Work out the finished part from the listing and answer in its coordinate system (mm). Give positions to 0.01 mm unless a question says otherwise; leave off trailing zeros. Write each loop counter-clockwise with the first axis right and the second up, starting at its lowest first coordinate (ties: lowest second). Pieces come first, ordered by that corner, then holes. Notation, with made-up numbers: (19.5, 29.5) -> (63.5, 29.5) arc R34 ccw to (63.5, 59.5) -> close; hole circle Ø11 at (2, -14.75). An arc over 180 degrees is marked (long way). Use a Markdown table: item, result. Add a question column.
Q1. Section C-C, the plane x = 107 is taken. Give the vertices of the cut face in (y, z), plus the area to 3 significant figures.
Q2. Section B-B, the plane y = 27.5 is taken. Give the vertices of the cut face in (x, z), plus the area to 3 significant figures.
Q3. Consider line 1 (Y direction, x = 18, z = 7.1); line 2 (Y direction, x = 52, z = 7.3); line 3 (X direction, y = 104, z = 8.55). Determine where each line is inside the solid, lowest interval first.
Q4. Section A-A, the plane z = 6.4 is taken. Give the vertices of the cut face in (x, y).
Q5. Each of these flat-tipped pins is pushed along its axis until it touches: pin 1 Ø1 at (y, z) = (102.5, 6) entering from -X; pin 2 Ø2.5 at (y, z) = (27.5, 7) entering from -X; pin 3 Ø5 at (x, y) = (155.28, 47.79) entering from +Z; pin 4 Ø2.5 at (x, z) = (6, 8) entering from -Y. Where does it stop, or does it pass through?
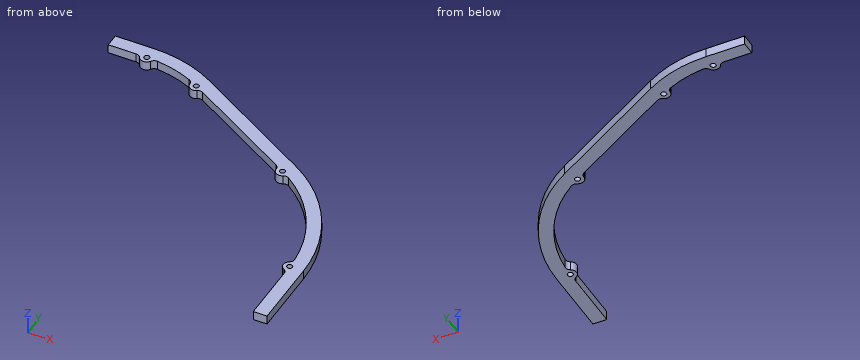
Solid Edge part; units mm, degrees
sketch "Sketch1" plane through (0.0007, 14.651, 5) normal (0, 0, 1) x (1, 0, 0)
  line L0 (-114.0407, 98.8093) -> (-57.2599, 131.5929)
  arc A0 (-54.1474, 131.5247) -> (-57.2599, 131.5929) centre (-55.7598, 128.9948) ccw
  arc A1 (-47.0142, 137.1861) -> (-48.7662, 134.4664) centre (-45.7662, 134.458) ccw
  arc A2 (-47.0142, 137.1861) -> (-26.9146, 142.5706) centre (-21.0226, 80.3698) cw
  arc A3 (-24.0376, 141.0909) -> (-26.9146, 142.5706) centre (-26.6317, 139.5839) ccw
  arc A4 (-15.245, 142.849) -> (-17.9063, 141.2336) centre (-15.245, 139.849) ccw
  line L1 (-15.245, 142.849) -> (15.2436, 142.849)
  arc A5 (17.905, 141.2336) -> (15.2436, 142.849) centre (15.2436, 139.849) ccw
  arc A6 (26.9132, 142.5696) -> (24.036, 141.0904) centre (26.6298, 139.583) ccw
  arc A7 (26.9132, 142.5696) -> (47.0027, 137.1869) centre (21.0099, 80.3561) cw
  arc A8 (48.7549, 134.4673) -> (47.0027, 137.1869) centre (45.7549, 134.4587) ccw
  arc A9 (57.2487, 131.5943) -> (54.1362, 131.526) centre (55.7487, 128.9962) ccw
  line L2 (57.2487, 131.5943) -> (114.0299, 98.8129)
  arc A10 (115.5271, 96.0833) -> (114.0299, 98.8129) centre (112.5299, 96.2148) ccw
  arc A11 (124.0003, 92.7805) -> (120.7849, 92.9052) centre (122.2944, 90.3127) ccw
  arc A12 (124.0003, 92.7805) -> (155.0355, 39.027) centre (82.7747, 33.1424) cw
  arc A13 (153.5358, 36.1799) -> (155.0355, 39.027) centre (152.0454, 38.7835) ccw
  arc A14 (155.2747, 27.3761) -> (153.6593, 30.0375) centre (152.2747, 27.3761) ccw
  line L3 (155.2747, 27.3761) -> (155.2747, -38.192)
  arc A15 (153.6593, -40.8534) -> (155.2747, -38.192) centre (152.2747, -38.192) ccw
  arc A16 (154.9954, -49.8615) -> (153.5161, -46.9844) centre (152.0088, -49.5782) ccw
  arc A17 (154.9954, -49.8615) -> (149.6134, -69.9554) centre (92.7533, -43.9583) cw
  arc A18 (146.8942, -71.7079) -> (149.6134, -69.9554) centre (146.8851, -68.7079) ccw
  arc A19 (144.0217, -80.2016) -> (143.9534, -77.0892) centre (141.4236, -78.7016) ccw
  line L4 (144.0217, -80.2016) -> (127.6444, -108.5679)
  arc A20 (122.7007, -116.5716) -> (122.8583, -113.3403) centre (120.256, -114.8329) ccw
  arc A21 (77.6703, -142.5696) -> (122.7007, -116.5716) centre (71.767, -80.3476) ccw
  arc A22 (74.7931, -141.0904) -> (77.6703, -142.5696) centre (77.3869, -139.583) ccw
  arc A23 (66.0007, -142.849) -> (68.6621, -141.2336) centre (66.0007, -139.849) ccw
  line L5 (5.7656, -142.849) -> (66.0007, -142.849)
  arc A24 (3.1042, -141.2336) -> (5.7656, -142.849) centre (5.7656, -139.849) ccw
  arc A25 (-5.767, -142.849) -> (-3.1056, -141.2336) centre (-5.767, -139.849) ccw
  line L6 (-66.0021, -142.849) -> (-5.767, -142.849)
  arc A26 (-68.6634, -141.2336) -> (-66.0021, -142.849) centre (-66.0021, -139.849) ccw
  arc A27 (-77.6716, -142.5694) -> (-74.7944, -141.0903) centre (-77.3881, -139.5828) ccw
  arc A28 (-122.6994, -116.5717) -> (-77.6716, -142.5694) centre (-71.7665, -80.349) ccw
  arc A29 (-122.857, -113.3404) -> (-122.6994, -116.5717) centre (-120.2547, -114.833) ccw
  arc A30 (-128.7762, -106.6053) -> (-126.0465, -108.1024) centre (-126.1781, -105.1053) ccw
  line L7 (-144.0218, -80.199) -> (-128.7762, -106.6053)
  arc A31 (-143.9535, -77.0865) -> (-144.0218, -80.199) centre (-141.4237, -78.699) ccw
  arc A32 (-149.6144, -69.9531) -> (-146.8949, -71.7053) centre (-146.8862, -68.7053) ccw
  arc A33 (-154.9987, -49.8585) -> (-149.6144, -69.9531) centre (-92.7672, -43.9523) ccw
  arc A34 (-153.5196, -46.9813) -> (-154.9987, -49.8585) centre (-152.0122, -49.5751) ccw
  arc A35 (-155.2786, -38.189) -> (-153.6631, -40.8503) centre (-152.2786, -38.1889) ccw
  line L8 (-155.2818, 27.3758) -> (-155.2786, -38.189)
  arc A36 (-153.6665, 30.0373) -> (-155.2818, 27.3758) centre (-152.2818, 27.376) ccw
  arc A37 (-155.0428, 39.0267) -> (-153.5432, 36.1796) centre (-152.0527, 38.7832) ccw
  arc A38 (-124.0109, 92.7765) -> (-155.0428, 39.0267) centre (-82.7847, 33.1421) ccw
  arc A39 (-120.7955, 92.9014) -> (-124.0109, 92.7765) centre (-122.3049, 90.3088) ccw
  arc A40 (-114.0407, 98.8093) -> (-115.5378, 96.0796) centre (-112.5406, 96.2112) ccw
  arc A41 (-48.7662, 134.4664) -> (-54.1474, 131.5247) centre (-52.2662, 134.4761) cw
  arc A42 (-17.9064, 141.2336) -> (-24.0377, 141.0909) centre (-21.0113, 142.849) cw
  arc A43 (24.036, 141.0904) -> (17.905, 141.2336) centre (21.0099, 142.849) cw
  arc A44 (54.1362, 131.526) -> (48.7549, 134.4673) centre (52.2549, 134.4774) cw
  arc A45 (120.7849, 92.9052) -> (115.5271, 96.0832) centre (119.0237, 95.9298) cw
  arc A46 (153.6593, 30.0375) -> (153.5358, 36.1799) centre (155.2747, 33.1424) cw
  arc A47 (153.5161, -46.9844) -> (153.6593, -40.8534) centre (155.2747, -43.9583) cw
  arc A48 (143.9534, -77.0891) -> (146.8942, -71.7079) centre (146.9048, -75.2079) cw
  arc A49 (122.8584, -113.3404) -> (127.6444, -108.5679) centre (125.8944, -111.599) cw
  arc A50 (68.6621, -141.2336) -> (74.7931, -141.0904) centre (71.767, -142.849) cw
  arc A51 (-3.1056, -141.2336) -> (3.1042, -141.2336) centre (-0.0007, -142.849) cw
  arc A52 (-74.7944, -141.0903) -> (-68.6635, -141.2336) centre (-71.7684, -142.849) cw
  arc A53 (-126.0466, -108.1024) -> (-122.857, -113.3404) centre (-125.8931, -111.599) cw
  arc A54 (-146.8949, -71.7053) -> (-143.9536, -77.0866) centre (-146.905, -75.2053) cw
  arc A55 (-153.6632, -40.8503) -> (-153.5196, -46.9813) centre (-155.2784, -43.9553) cw
  arc A56 (-153.5432, 36.1796) -> (-153.6665, 30.0373) centre (-155.2821, 33.1421) cw
  arc A57 (-115.5377, 96.0796) -> (-120.7955, 92.9014) centre (-119.0344, 95.926) cw
  line L9 (-56.0166, 140.971) -> (-122.7845, 102.4212)
  arc A58 (-162.7821, 33.1421) -> (-122.7845, 102.4212) centre (-82.7847, 33.1421) cw
  line L10 (-162.7821, 33.1421) -> (-162.7784, -43.9553)
  arc A59 (-162.7784, -43.9553) -> (-153.4002, -78.9553) centre (-92.7784, -43.9553) ccw
  line L11 (-132.3882, -115.349) -> (-153.4002, -78.9553)
  arc A60 (-132.3882, -115.349) -> (-71.7683, -150.349) centre (-71.7665, -80.349) ccw
  line L12 (71.767, -150.349) -> (-71.7683, -150.349)
  arc A61 (71.767, -150.349) -> (132.3896, -115.349) centre (71.7678, -80.349) ccw
  line L13 (132.3896, -115.349) -> (153.4002, -78.9576)
  arc A62 (162.7747, -43.9583) -> (153.4002, -78.9576) centre (92.791, -43.9684) cw
  line L14 (162.7747, 33.1424) -> (162.7747, -43.9583)
  arc A63 (122.7736, 102.4251) -> (162.7747, 33.1424) centre (82.7747, 33.1424) cw
  line L15 (56.0045, 140.9728) -> (122.7736, 102.4251)
  arc A64 (21.0099, 150.349) -> (56.0045, 140.9728) centre (21.008, 80.349) cw
  line L16 (-21.0112, 150.349) -> (21.0099, 150.349)
  arc A65 (-32.5074, 149.4015) -> (-21.0112, 150.349) centre (-20.997, 79.961) cw
  arc A66 (-44.641, 146.2432) -> (-32.5074, 149.4015) centre (-21.0122, 80.3518) cw
  arc A67 (-56.0166, 140.971) -> (-44.641, 146.2432) centre (-21.0122, 80.3518) cw
  circle A68 centre (-71.7683, -142.849) radius 1.5
  circle A69 centre (-0.0007, -142.849) radius 1.5
  circle A70 centre (-125.893, -111.599) radius 1.5
  circle A71 centre (-146.905, -75.2053) radius 1.5
  circle A72 centre (-155.2784, -43.9553) radius 1.5
  circle A73 centre (-155.2821, 33.1421) radius 1.5
  circle A74 centre (-119.0344, 95.9261) radius 1.5
  circle A75 centre (-52.2662, 134.4761) radius 1.5
  circle A76 centre (-21.0112, 142.849) radius 1.5
  circle A77 centre (21.0099, 142.849) radius 1.5
  circle A78 centre (52.2549, 134.4774) radius 1.5
  circle A79 centre (119.0237, 95.9298) radius 1.5
  circle A80 centre (155.2747, 33.1424) radius 1.5
  circle A81 centre (155.2747, -43.9583) radius 1.5
  circle A82 centre (146.9048, -75.2079) radius 1.5
  circle A83 centre (125.8944, -111.599) radius 1.5
  circle A84 centre (71.767, -142.849) radius 1.5
extrude "ExtrudedProtrusion_7" add sketch "Sketch1" along normal blind 5
sketch "Sketch2" plane through (-0.003, 14.651, 10) normal (0, 0, 1) x (1, 0, 0)
  line L0 (-170.0115, -5.4066) -> (169.0999, -5.4066)
  line L1 (169.0999, -5.4066) -> (169.0999, -159.984)
  line L2 (169.0999, -159.984) -> (-170.0115, -159.984)
  line L3 (-170.0115, -159.984) -> (-170.0115, -5.4066)
extrude "Cutout1" cut sketch "Sketch2" against normal up to next
sketch "Sketch3" plane through (-0.003, 87.1222, 10) normal (0, 0, 1) x (0.866, -0.5, 0)
  line L0 (-35.1853, 60.951) -> (-42.5637, 73.7312)
  line L1 (-42.5637, 73.7312) -> (-202.1881, -18.4247)
  line L2 (-202.1881, -18.4247) -> (-113.6218, -171.8315)
  line L3 (-113.6218, -171.8315) -> (46.0026, -79.6757)
  line L4 (-35.1853, 60.951) -> (46.0026, -79.6757)
extrude "Cutout2" cut sketch "Sketch3" against normal up to next
properties material "Polycarbonate"
Result set:
| question | item | result |
|---|---|---|
| 1 | outline | (117.52, 5) -> (126.18, 5) -> (126.18, 10) -> (117.52, 10) -> close |
| 1 | area | 43.3 mm2 |
| 2 | outline | (155.28, 5) -> (162.78, 5) -> (162.78, 10) -> (155.28, 10) -> close |
| 2 | area | 37.5 mm2 |
| 3 | line 1 | y = 155.71 to 165 |
| 3 | line 2 | y = 145.64 to 147.65, 150.61 to 157.77 |
| 3 | line 3 | x = 128.57 to 139.7 |
| 4 | outline | (0, 157.5) -> (15.24, 157.5) arc R3 cw to (17.91, 155.88) arc R3.5 ccw to (24.04, 155.74) arc R3 cw to (26.91, 157.22) arc R62.49 cw to (47, 151.84) arc R3 cw to (48.76, 149.12) arc R3.5 ccw to (54.14, 146.18) arc R3 cw to (57.25, 146.25) -> (114.03, 113.46) arc R3 cw to (115.53, 110.73) arc R3.5 ccw to (120.79, 107.56) arc R3 cw to (124, 107.43) arc R72.5 cw to (155.04, 53.68) arc R3 cw to (153.54, 50.83) arc R3.5 ccw to (153.66, 44.69) arc R3 cw to (155.28, 42.03) -> (155.28, 9.24) -> (162.78, 9.24) -> (162.78, 47.79) arc R80 ccw to (122.77, 117.08) -> (56.01, 155.62) arc R70 ccw to (21.01, 165) -> (0, 165) -> close; hole circle Ø3 at (21.01, 157.5); hole circle Ø3 at (52.26, 149.13); hole circle Ø3 at (119.02, 110.58); hole circle Ø3 at (155.28, 47.79) |
| 5 | pin 1 | stops at x = 129.77 |
| 5 | pin 2 | stops at x = 155.28 |
| 5 | pin 3 | stops at z = 10 |
| 5 | pin 4 | stops at y = 157.5 |
